```python
from build123d import *

# Parameters (mm, degrees)
CROQUIS2_R                = 4.7625
SALIENTE_EXTRUIR1_DEPTH   = 36.5125
CHAFL_N1_SIZE             = 0.396875
CROQUIS4_R                = 2.4892
CLEARANCE_HOLE_DEPTH      = 37.5125
CLEARANCE_HOLE_DEPTH_BACK = 37.5125


with BuildPart() as part:
    # Croquis2 → Saliente-Extruir1 (new body, symmetric)
    with BuildSketch(Plane(origin=(0, 0, 0), x_dir=(1, 0, 0), z_dir=(0, 1, 0))):
        Circle(CROQUIS2_R)
    extrude(amount=SALIENTE_EXTRUIR1_DEPTH, both=True)

    # Chafl_n1
    chafl_n1_edges = [part.edges().sort_by_distance(p)[0] for p in [
        (-4.7625, -36.5125, 0),
        (-4.7625, 36.5125, 0),
    ]]
    chamfer(chafl_n1_edges, length=CHAFL_N1_SIZE)

    # Croquis4 → Clearance Hole (cut, two sides)
    with BuildSketch(Plane(origin=(0, 0, 0), x_dir=(1, 0, 0), z_dir=(0, 1, 0))) as clearance_hole_sk:
        Circle(CROQUIS4_R)
    extrude(amount=CLEARANCE_HOLE_DEPTH, mode=Mode.SUBTRACT)
    extrude(clearance_hole_sk.sketch, amount=-CLEARANCE_HOLE_DEPTH_BACK, mode=Mode.SUBTRACT)


solid = part.part
```
For this review, take the finished solid that the model builds, in its own axes (mm). Coordinates: 2 decimals unless noted, no trailing zeros. Loops run counter-clockwise (first coordinate to the right, second up) from the corner with the lowest first, then second, coordinate; pieces in that order, holes last.
1. For line 1 (X direction, y = 5, z = 0); line 2 (Z direction, x = 2, y = 7.5), list the stretches that pass through material, from the lowest coordinate up.
2. Add section C-C, the plane y = -10. Give the boundary of the cut face in (x, z) (1 decimal).
3. Insertion check: P1, Ø3, axis at x = -1, y = -4, coming from the -Z side; P2, Ø1, axis at y = -13.5, z = -1, coming from the +X side. Each pin has a flat end and moves straight along its axis. Give the tip position at first contact, or say it passes through.
4. Add section A-A, the plane x = 0. Give the boundary of the cut face in (y, z), then the cut area to 3 significant figures.
5. Add section B-B, the plane z = 0. Give the boundary of the cut face in (x, y), then the cut area to 3 significant figures.
6. Mouldability with a two-part tool opening along Z and no side actions: class faces 1 (the cylindrical face through (-3.78, 0.51, 2.9)), 2 (the cylindrical face through (2.374, 0.511, -0.748)), 3 (the flat face through (2, -36.512, 2)) as +Z half, -Z half, draft (parallel to the pull), parting line (faces both ways), or undercut.
Result:
1. line 1: x = -4.76 to -2.49, 2.49 to 4.76
1. line 2: z = -4.32 to -1.48, 1.48 to 4.32
2. outline: circle Ø9.5 at (0, 0); hole circle Ø5 at (0, 0)
3. P1: stops at z = -4.76
3. P2: stops at x = 4.74
4. outline: (-36.51, -4.37) - (-36.12, -4.76) - (36.12, -4.76) - (36.51, -4.37) - (36.51, -2.49) - (-36.51, -2.49) - close; (-36.51, 2.49) - (36.51, 2.49) - (36.51, 4.37) - (36.12, 4.76) - (-36.12, 4.76) - (-36.51, 4.37) - close
4. area: 332 mm2
5. outline: (-4.76, -36.12) - (-4.37, -36.51) - (-2.49, -36.51) - (-2.49, 36.51) - (-4.37, 36.51) - (-4.76, 36.12) - close; (2.49, -36.51) - (4.37, -36.51) - (4.76, -36.12) - (4.76, 36.12) - (4.37, 36.51) - (2.49, 36.51) - close
5. area: 332 mm2
6. face 1: parting line
6. face 2: undercut
6. face 3: draft
